from build123d import *

# Parameters (mm, degrees)
SKETCH_1_W         = 20
SKETCH_1_H         = 8
EXTRUDE_1_DEPTH    = 6
HOLE_WIZARD_M3_1_D = 2.5
HOLE_WIZARD_M3_2_D = 2.5
CHAMFER_1_SIZE     = 0.3


with BuildPart() as part:
    # 草图1 → 凸台-拉伸1 (new body)
    with BuildSketch(Plane(origin=(0, 0, 0), x_dir=(1, 0, 0), z_dir=(0, 1, 0))):
        Rectangle(SKETCH_1_W, SKETCH_1_H)
    extrude(amount=EXTRUDE_1_DEPTH)

    # M3 螺纹孔1 (through all)
    with Locations(Plane(origin=(6.5, 3, -4), x_dir=(-1, 0, 0), z_dir=(0, 0, -1))):
        with Locations((0, 0), (13, 0)):
            Hole(HOLE_WIZARD_M3_1_D / 2)

    # M3 螺纹孔2 (through all)
    with Locations(Plane.ZX.offset(6)):
        with Locations((0, 0)):
            Hole(HOLE_WIZARD_M3_2_D / 2)

    # 倒角1
    chamfer_1_edges = [part.edges().sort_by_distance(p)[0] for p in [
        (-10, 6, 0),
        (0, 6, 4),
        (10, 6, 0),
        (0, 0, 4),
        (-10, 0, 0),
        (0, 0, -4),
        (10, 0, 0),
        (10, 3, 4),
        (-10, 3, 4),
        (-10, 3, -4),
        (10, 3, -4),
        (0, 6, -4),
    ]]
    chamfer(chamfer_1_edges, length=CHAMFER_1_SIZE)


solid = part.part
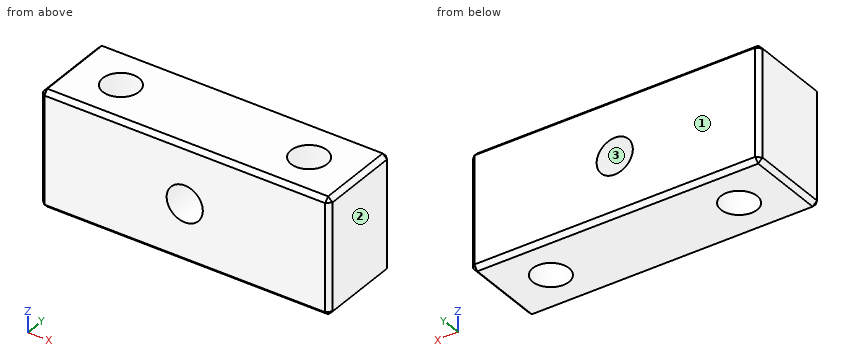
Read the model definition and answer for the solid it produces. Units are mm, in the model's axes. Face numbers are marked on the shaded views. Round coordinates to 2 decimals unless told otherwise and drop trailing zeros. Order: outer loops, then holes, each group sorted by start corner. A loop starts at its lowest first (then second) coordinate and runs counter-clockwise, first axis right, second up.
1) The part is cut by section D-D on z = -3. Write down the section's boundary in (x, y).
2) A flat-ended cylindrical pin translates along its axis: pin 1 (1.5 mm diameter, centred on x = -6.5, y = 3, fed in from +Z). Find the tip coordinate at first contact, or state that the pin passes through.
3) The part is cut by section C-C on x = -6.5. Write down the section's boundary in (y, z).
4) The part is cut by section A-A on z = 0. Write down the section's boundary in (x, y), plus the area to 3 significant figures.
5) The part is cut by section B-B on y = 3. Write down the section's boundary in (x, z).
6) The mould has two halves that part along X. Classify the marked faces 1, 2 and 3: released by +X, released by -X, zero draft, split by the parting line, or undercut.
7) Straight lines are drawn through the part: L1, parallel to X at y = 2.75, z = -2.25; L2, parallel to X at y = 2.25, z = 2; L3, parallel to Y at x = 6.5, z = 0. For each, find the intervals that lie inside material, in ascending order.
Resolved:
1. outline: (-10, 0.3) - (-9.7, 0) - (9.7, 0) - (10, 0.3) - (10, 5.7) - (9.7, 6) - (-9.7, 6) - (-10, 5.7) - close; hole circle Ø2.5 at (-6.5, 3); hole circle Ø2.5 at (6.5, 3)
2. pin 1: passes through
3. outline: (0, -3.7) - (0.3, -4) - (1.75, -4) - (1.75, 4) - (0.3, 4) - (0, 3.7) - close; (4.25, -4) - (5.7, -4) - (6, -3.7) - (6, 3.7) - (5.7, 4) - (4.25, 4) - close
4. outline: (-10, 0.3) - (-9.7, 0) - (-1.25, 0) - (-1.25, 6) - (-9.7, 6) - (-10, 5.7) - close; (1.25, 0) - (9.7, 0) - (10, 0.3) - (10, 5.7) - (9.7, 6) - (1.25, 6) - close; hole circle Ø2.5 at (-6.5, 3); hole circle Ø2.5 at (6.5, 3)
4. area: 95.0 mm2
5. outline: (-10, -3.7) - (-9.7, -4) - (-7.75, -4) - (-7.75, 4) - (-9.7, 4) - (-10, 3.7) - close; (-5.25, -4) - (5.25, -4) - (5.25, 4) - (-5.25, 4) - close; (7.75, -4) - (9.7, -4) - (10, -3.7) - (10, 3.7) - (9.7, 4) - (7.75, 4) - close; hole circle Ø2.5 at (0, 0)
6. face 1: zero draft
6. face 2: released by +X
6. face 3: undercut
7. L1: x = -10 to -7.72, -5.28 to 5.28, 7.72 to 10
7. L2: x = -10 to -7.5, -5.5 to 5.5, 7.5 to 10
7. L3: y = 0 to 1.75, 4.25 to 6
